Part model, mm, in its own coordinate system. Coordinates: 2 decimals unless noted, no trailing zeros.
1) Pin check, flat tip, straight feed: pin 1 Ø7.5 at (x, z) = (-138.89, 482.45) entering from +Y. Stop position of the tip, or through.
2) Wall check: L1, parallel to Z at x = -15, y = 2.75; L2, parallel to X at y = 10, z = 535.5. Give the ranges that are in metal, low to high.
3) Mould opens along X. For faces 1 (the flat face through (0, 6, 283)), 2 (the flat face through (-77, 6, 558.8)), 3 (the flat face through (-152.4, 6, 283)), 4 (the cylindrical face through (-12.138, 6.261, 82.546)) say: +X half, -X half, draft (parallel to the pull), parting line (faces both ways), or undercut.
```python
from build123d import *

# Parameters (mm, degrees)
SKETCH1_W           = 152.4
SKETCH1_H           = 558.8
BOSS_EXTRUDE1_DEPTH = 12.7
CUT_EXTRUDE1_REACH  = 14.7
SKETCH2_R           = 6.35


with BuildPart() as part:
    # Sketch1 → Boss-Extrude1 (new body)
    with BuildSketch(Plane(origin=(0, 0, 0), x_dir=(1, 0, 0), z_dir=(0, 1, 0))):
        with Locations((-76.2, -279.4)):
            Rectangle(SKETCH1_W, SKETCH1_H)
    extrude(amount=BOSS_EXTRUDE1_DEPTH)

    # Sketch2 → Cut-Extrude1 (cut, up to next)
    with BuildSketch(Plane(origin=(0, 0, 0), x_dir=(-1, 0, 0), z_dir=(0, -1, 0)), mode=Mode.PRIVATE) as cut_extrude1_sk1:
        with Locations((13.51432586, -25.547353246)):
            Circle(SKETCH2_R)
    cut_extrude1_tool1 = extrude(cut_extrude1_sk1.sketch, amount=-CUT_EXTRUDE1_REACH, mode=Mode.PRIVATE) & part.part
    add(cut_extrude1_tool1.solids().sort_by_distance((-13.514326, 0, 25.547353))[0], mode=Mode.SUBTRACT)
    # Sketch2 → Cut-Extrude1 (cut, up to next)
    with BuildSketch(Plane(origin=(0, 0, 0), x_dir=(-1, 0, 0), z_dir=(0, -1, 0)), mode=Mode.PRIVATE) as cut_extrude1_sk2:
        with Locations((13.51432586, -76.347353246)):
            Circle(SKETCH2_R)
    cut_extrude1_tool2 = extrude(cut_extrude1_sk2.sketch, amount=-CUT_EXTRUDE1_REACH, mode=Mode.PRIVATE) & part.part
    add(cut_extrude1_tool2.solids().sort_by_distance((-13.514326, 0, 76.347353))[0], mode=Mode.SUBTRACT)
    # Sketch2 → Cut-Extrude1 (cut, up to next)
    with BuildSketch(Plane(origin=(0, 0, 0), x_dir=(-1, 0, 0), z_dir=(0, -1, 0)), mode=Mode.PRIVATE) as cut_extrude1_sk3:
        with Locations((13.51432586, -482.452646754)):
            Circle(SKETCH2_R)
    cut_extrude1_tool3 = extrude(cut_extrude1_sk3.sketch, amount=-CUT_EXTRUDE1_REACH, mode=Mode.PRIVATE) & part.part
    add(cut_extrude1_tool3.solids().sort_by_distance((-13.514326, 0, 482.452647))[0], mode=Mode.SUBTRACT)
    # Sketch2 → Cut-Extrude1 (cut, up to next)
    with BuildSketch(Plane(origin=(0, 0, 0), x_dir=(-1, 0, 0), z_dir=(0, -1, 0)), mode=Mode.PRIVATE) as cut_extrude1_sk4:
        with Locations((13.51432586, -533.252646754)):
            Circle(SKETCH2_R)
    cut_extrude1_tool4 = extrude(cut_extrude1_sk4.sketch, amount=-CUT_EXTRUDE1_REACH, mode=Mode.PRIVATE) & part.part
    add(cut_extrude1_tool4.solids().sort_by_distance((-13.514326, 0, 533.252647))[0], mode=Mode.SUBTRACT)
    # Sketch2 → Cut-Extrude1 (cut, up to next)
    with BuildSketch(Plane(origin=(0, 0, 0), x_dir=(-1, 0, 0), z_dir=(0, -1, 0)), mode=Mode.PRIVATE) as cut_extrude1_sk5:
        with Locations((138.88567414, -76.347353246)):
            Circle(SKETCH2_R)
    cut_extrude1_tool5 = extrude(cut_extrude1_sk5.sketch, amount=-CUT_EXTRUDE1_REACH, mode=Mode.PRIVATE) & part.part
    add(cut_extrude1_tool5.solids().sort_by_distance((-138.885674, 0, 76.347353))[0], mode=Mode.SUBTRACT)
    # Sketch2 → Cut-Extrude1 (cut, up to next)
    with BuildSketch(Plane(origin=(0, 0, 0), x_dir=(-1, 0, 0), z_dir=(0, -1, 0)), mode=Mode.PRIVATE) as cut_extrude1_sk6:
        with Locations((138.88567414, -25.547353246)):
            Circle(SKETCH2_R)
    cut_extrude1_tool6 = extrude(cut_extrude1_sk6.sketch, amount=-CUT_EXTRUDE1_REACH, mode=Mode.PRIVATE) & part.part
    add(cut_extrude1_tool6.solids().sort_by_distance((-138.885674, 0, 25.547353))[0], mode=Mode.SUBTRACT)
    # Sketch2 → Cut-Extrude1 (cut, up to next)
    with BuildSketch(Plane(origin=(0, 0, 0), x_dir=(-1, 0, 0), z_dir=(0, -1, 0)), mode=Mode.PRIVATE) as cut_extrude1_sk7:
        with Locations((138.88567414, -482.452646754)):
            Circle(SKETCH2_R)
    cut_extrude1_tool7 = extrude(cut_extrude1_sk7.sketch, amount=-CUT_EXTRUDE1_REACH, mode=Mode.PRIVATE) & part.part
    add(cut_extrude1_tool7.solids().sort_by_distance((-138.885674, 0, 482.452647))[0], mode=Mode.SUBTRACT)
    # Sketch2 → Cut-Extrude1 (cut, up to next)
    with BuildSketch(Plane(origin=(0, 0, 0), x_dir=(-1, 0, 0), z_dir=(0, -1, 0)), mode=Mode.PRIVATE) as cut_extrude1_sk8:
        with Locations((138.88567414, -533.252646754)):
            Circle(SKETCH2_R)
    cut_extrude1_tool8 = extrude(cut_extrude1_sk8.sketch, amount=-CUT_EXTRUDE1_REACH, mode=Mode.PRIVATE) & part.part
    add(cut_extrude1_tool8.solids().sort_by_distance((-138.885674, 0, 533.252647))[0], mode=Mode.SUBTRACT)


solid = part.part
```
Geometry check:
1. pin 1: passes through
2. L1: z = 0 to 19.37, 31.72 to 70.17, 82.52 to 476.28, 488.63 to 527.08, 539.43 to 558.8
2. L2: x = -152.4 to -144.82, -132.95 to -19.45, -7.58 to 0
3. face 1: +X half
3. face 2: draft
3. face 3: -X half
3. face 4: undercut
